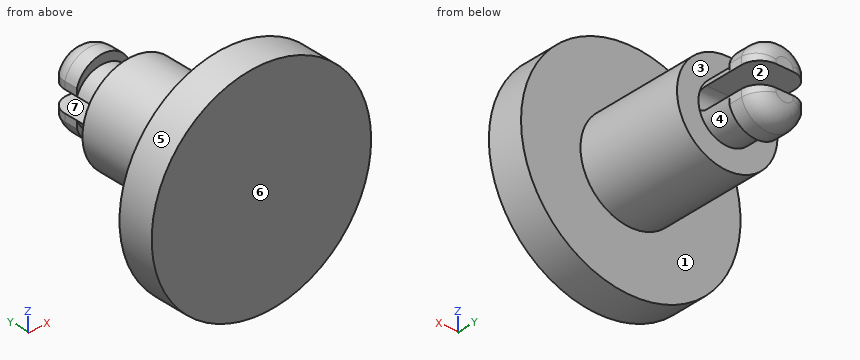
Autodesk Inventor part; units mm, degrees
ref_plane "YZ Plane" through (0, 0, 0) normal (1, 0, 0) x (0, 1, 0)
ref_plane "XZ Plane" through (0, 0, 0) normal (0, 1, 0) x (-1, 0, 0)
ref_plane "XY Plane" through (0, 0, 0) normal (0, 0, 1) x (1, 0, 0)
sketch "Sketch1" plane through (0, 0, 0) normal (0, 1, 0) x (-1, 0, 0)
  circle A0 centre (43.0199, -7.0958) radius 2.75
  circle A1 centre (-31.8801, -7.0958) radius 2.75
  circle A2 centre (44.3199, 41.1042) radius 2.75
  circle A3 centre (-38.2801, 41.1042) radius 2.75
  line L0 (58.8879, -10.055) -> (-40.7911, -10.055) construction
  line L1 (-40.7911, -10.055) -> (-40.7911, 44.0634) construction
  line L2 (-40.7911, 44.0634) -> (58.8879, 44.0634) construction
  line L3 (58.8879, 44.0634) -> (58.8879, -10.055) construction
  line L4 (43.0199, -7.0958) -> (43.0199, -10.055)
  line L5 (44.3199, 41.1042) -> (44.3199, 44.0634)
  line L6 (47.0699, -9.8458) -> (-41.0301, -9.8458)
  line L7 (-41.0301, -9.8458) -> (-41.0301, 43.8542)
  line L8 (-41.0301, 43.8542) -> (47.0699, 43.8542)
  line L9 (47.0699, 43.8542) -> (47.0699, -9.8458)
  dimension "d0" = 5.5
  dimension "d1" = 74.9
  dimension "d2" = 1.3
  dimension "d3" = 48.2
  dimension "d5" = 82.6
  dimension "d9" = 15.868
  dimension "d10" = 54.1184
  dimension "d11" = 99.679
extrude "Extrusion2" add sketch "Sketch1" along normal blind 6 contours A0
sketch "Sketch4" plane through (-43.0199, 6, -7.0958) normal (0, 1, 0) x (1, 0, 0)
  circle A0 centre (0, 0) radius 2.75
  circle A1 centre (0, 0) radius 1.575
  point P0 (43.0199, -7.0958)
  dimension "d24" = 3.15
extrude "Extrusion3" add sketch "Sketch4" along normal blind 1.8 contours A1
sketch "Sketch5" plane through (-43.0199, 7.8, -7.0958) normal (0, 1, 0) x (1, 0, 0)
  line L0 (-1.575, -0.575) -> (1.575, -0.575)
  line L1 (1.575, -0.575) -> (1.575, 0.575)
  line L2 (1.575, 0.575) -> (-1.575, 0.575)
  line L3 (-1.575, 0.575) -> (-1.575, -0.575)
  line L4 (-1.575, -0.575) -> (1.575, 0.575) construction
  line L5 (1.575, -0.575) -> (-1.575, 0.575) construction
  circle A0 centre (0, 0) radius 1.575
  point P0 (43.0199, -7.0958)
  point P1 (-1.4663, -0.575)
  point P2 (1.4663, -0.575)
  point P3 (1.4663, 0.575)
  point P4 (-1.4663, 0.575)
  dimension "d27" = 1
extrude "Extrusion4" cut sketch "Sketch5" against normal blind 6 contours A0 L2 L0
sketch "Sketch6" plane through (-43.0199, 7.8, -7.0958) normal (0, 1, 0) x (1, 0, 0)
  arc A0 (1.4663, 0.575) -> (-1.4663, 0.575) centre (0, 0) ccw construction
  line L0 (-1.4663, 0.575) -> (-1.4663, 0.975)
  line L1 (-1.4663, 0.575) -> (1.4663, 0.575)
  line L2 (1.4663, 0.575) -> (1.4663, 0.975)
  arc A1 (1.4663, 0.975) -> (-1.4663, 0.975) centre (0, 0.5477) ccw
  arc A2 (-1.4663, 0.575) -> (-1.4663, -0.575) centre (0, 0) ccw construction
  line L3 (-1.575, 0) -> (1.575, 0) construction
  arc A3 (1.4663, -0.575) -> (1.4663, 0.575) centre (0, 0) ccw construction
  line L4 (-1.4663, -0.575) -> (-1.4663, -0.975)
  line L5 (-1.4663, -0.575) -> (1.4663, -0.575)
  line L6 (1.4663, -0.575) -> (1.4663, -0.975)
  arc A4 (-1.4663, -0.975) -> (1.4663, -0.975) centre (0, -0.5477) ccw
  point P0 (43.0199, -7.0958)
  point P1 (0, 1.575)
  point P2 (0, 2.075)
  dimension "d30" = 0.4
  dimension "d31" = 0.4
  dimension "d32" = 0.5
extrude "Extrusion5" add sketch "Sketch6" along normal blind 1.75
fillet "Fillet1" radius 1 6 edges at (-44.4862, 9.55, -6.3208) (-41.5537, 9.55, -6.3208) (-43.0199, 9.55, -5.0208) (-41.5537, 9.55, -7.8708) (-44.4862, 9.55, -7.8708) (-43.0199, 9.55, -9.1708)
sketch "Sketch7" plane through (-43.0199, 1.8, -7.0958) normal (0, 1, 0) x (1, 0, 0)
  line L0 (1.4663, -0.575) -> (-1.4663, -0.575)
  arc A0 (1.4663, -0.575) -> (1.4663, 0.575) centre (0, 0) ccw
  line L1 (-1.4663, 0.575) -> (1.4663, 0.575)
  arc A1 (-1.4663, 0.575) -> (-1.4663, -0.575) centre (0, 0) ccw
  point P0 (43.0199, -7.0958)
extrude "Extrusion6" add sketch "Sketch7" along normal blind 4
fillet "Fillet2" radius 0.575 2 edges at (-43.0199, 5.8, -7.6708) (-43.0199, 5.8, -6.5208)
sketch "Sketch16" plane through (-43.0199, 0, -7.0958) normal (0, -1, 0) x (1, 0, 0)
  circle A0 centre (0, 0) radius 6
  point P0 (43.0199, 7.0958)
  dimension "d56" = 12
extrude "Extrusion9" add sketch "Sketch16" along normal blind 2
properties part number "arduino_mega_standoffs_retention-clips_single"
Check sheet for the modelled part. Datum: model origin and axes. Units: mm. Face numbers are marked on the shaded views. A direction names the side the tool comes from. Round coordinates to 2 decimals unless told otherwise and drop trailing zeros. Loops run counter-clockwise (first coordinate to the right, second up) from the corner with the lowest first, then second, coordinate; pieces in that order, holes last. Notation, with made-up numbers: (-19, 23) -> (-13, 23) arc R28 cw to (-13, 58) -> close; hole circle Ø7 at (-1.75, 36.25). An arc over 180 degrees is marked (long way). Write item = value, one per line. Start each with the question number.
1) Gauge pin test, flat ends, axial feed: pin 1 Ø3 at (x, y) = (-43.5, 8) entering from -Z; pin 2 Ø3 at (x, z) = (-44.5, -6.5) entering from +Y; pin 3 Ø1.5 at (y, z) = (7.5, -8.5) entering from -X; pin 4 Ø3 at (x, y) = (-42.5, 8.5) entering from +Z. Record the tip position at first contact, or that the pin passes through.
2) Thickness scan on probe 1 along Y at (x, z) = (-42.75, -4.25); probe 2 along Z at (x, y) = (-42, 6.75); probe 3 along Y at (x, z) = (-45.25, -5.75). Record the ranges inside material, lowest first.
3) Release check for a two-part mould opening along Z. For the marked faces 4, 5, 6 and 7 record: released by +Z, released by -Z, zero draft, split by the parting line, or undercut.
4) Sectioned sample at D-D, the plane y = 1. Record the cut outline in (x, z), plus the area to 3 significant figures.
5) Sectioned sample at A-A, the plane x = -45.5. Record the cut outline in (y, z), plus the area to 3 significant figures.
6) Sectioned sample at B-B, the plane z = -9.5. Record the cut outline in (x, y), plus the area to 3 significant figures.
7) Set-up check for the marked faces 1, 2 and 3: record each of +Z, -Z, +X, -X, +Y, -Y from which the full face is reachable in a straight line by a thin tool's end or side.
8) Sectioned sample at C-C, the plane y = 6.75. Record the cut outline in (x, z) (3 decimals).
Results are:
q1.pin_1 = -9.17
q1.pin_2 = 9.55
q1.pin_3 = -44.49
q1.pin_4 = -5.02
q2.probe_1 = -2 to 0
q2.probe_2 = -8.3 to -7.67, -6.52 to -5.9
q2.probe_3 = -2 to 6
q3.face_4 = released by -Z
q3.face_5 = split by the parting line
q3.face_6 = zero draft
q3.face_7 = undercut
q4.outline = circle Ø5.5 at (-43.02, -7.1)
q4.area = 23.8 mm^2
q5.outline = (-2, -12.56) -> (0, -12.56) -> (0, -8.28) -> (6, -8.28) -> (6, -5.91) -> (0, -5.91) -> (0, -1.63) -> (-2, -1.63) -> close
q5.area = 36.1 mm^2
q6.outline = (-48.52, -2) -> (-37.52, -2) -> (-37.52, 0) -> (-41.68, 0) -> (-41.68, 6) -> (-44.35, 6) -> (-44.35, 0) -> (-48.52, 0) -> close
q6.area = 38.0 mm^2
q7.face_1 = +Y
q7.face_2 = +X, -X, +Y
q7.face_3 = none
q8.outline = (-44.486, -7.671) arc R1.575 ccw to (-41.554, -7.671) -> close; (-44.486, -6.521) -> (-41.554, -6.521) arc R1.575 ccw to start
